CAD build for the part. Positions are in the model's coordinates, mm. Face numbers are marked on the shaded views. Round coordinates to 2 decimals unless told otherwise and drop trailing zeros. Order: outer loops, then holes, each group sorted by start corner. A loop starts at its lowest first (then second) coordinate and runs counter-clockwise, first axis right, second up. Notation, with made-up numbers: M 80,-39 L 137,-39 A21 cw 137,-13 Z; hole C 0,87.25 d6. An arc over 180 degrees is marked long. Answer as a JSON object with one key per item and string values. Group by question number.
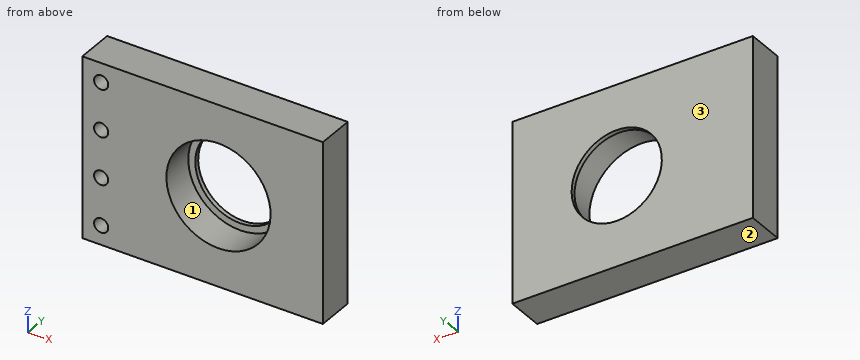
```python
from build123d import *

# Parameters (mm, degrees)
SKETCH1_W          = 50.8
SKETCH1_H          = 38.1
BODY_DEPTH         = 7.9375
SKETCH_1_R         = 9.525
THRU_HOLE_DEPTH    = 33.727150903
SKETCH4_R          = 10.9982
BEARING_BORE_DEPTH = 7.0104
SKETCH5_R          = 1.4986
DOWEL_HOLES_DEPTH  = 6.5


with BuildPart() as part:
    # Sketch1 → Body (new body)
    with BuildSketch(Plane(origin=(0, 0, 0), x_dir=(1, 0, 0), z_dir=(0, 1, 0))):
        Rectangle(SKETCH1_W, SKETCH1_H)
    extrude(amount=BODY_DEPTH)

    # Sketch 1 → Thru Hole (cut, through all)
    with BuildSketch(Plane.XZ):
        with Locations(Location((3.3528, 0, 0), (0, 0, 270))):
            Circle(SKETCH_1_R)
    extrude(amount=-THRU_HOLE_DEPTH, mode=Mode.SUBTRACT)

    # Sketch4 → Bearing Bore (cut)
    with BuildSketch(Plane.XZ):
        with Locations(Location((3.3528, 0, 0), (0, 0, 270))):
            Circle(SKETCH4_R)
    extrude(amount=-BEARING_BORE_DEPTH, mode=Mode.SUBTRACT)

    # Sketch5 → Dowel Holes (cut)
    with BuildSketch(Plane.XZ):
        with Locations(Location((-21.4249, 14.986, 0), (0, 0, 270))):
            Circle(SKETCH5_R)
        with Locations(Location((-21.4249, 4.995333333, 0), (0, 0, 270))):
            Circle(SKETCH5_R)
        with Locations(Location((-21.4249, -14.986, 0), (0, 0, 270))):
            Circle(SKETCH5_R)
        with Locations(Location((-21.4249, -4.995333333, 0), (0, 0, 270))):
            Circle(SKETCH5_R)
    extrude(amount=-DOWEL_HOLES_DEPTH, mode=Mode.SUBTRACT)


solid = part.part
```
Item 1: Cut at B-B, the plane x = 2. Give the cut face in (y, z).
Item 2: Two-plate mould, pull along Z, no slides. Class the marked faces 1, 2 and 3: +Z half, -Z half, draft (parallel to the pull), parting line (faces both ways), or undercut.
Item 3: Cut at D-D, the plane z = -14. Give the cut face in (x, y), and give its area (3 significant figures).
Item 4: Flat gauge pins, fed straight in: pin 1 Ø1.5 at (x, z) = (-21, -5.5) entering from -Y; pin 2 Ø2 at (x, z) = (13, 2) entering from -Y. Where does each tip first touch, or does it go through?
Item 5: Cut at A-A, the plane z = 0. Give the cut face in (x, y).
Item 6: Cut at C-C, the plane y = 2. Give the cut face in (x, z).
Item 7: Drill centre lines: line 1 (X direction, y = 1, z = -15); line 2 (X direction, y = 6.25, z = -4); line 3 (X direction, y = 1.25, z = -2). Where is each one in solid material? Low to high. Write a range as [from, to].
Response values:
{
 "1": {"outline": "M 0,-19.05 L 7.94,-19.05 L 7.94,-9.43 L 7.01,-9.43 L 7.01,-10.91 L 0,-10.91 Z; M 0,10.91 L 7.01,10.91 L 7.01,9.43 L 7.94,9.43 L 7.94,19.05 L 0,19.05 Z"},
 "2": {"face 1": "undercut", "face 2": "-Z half", "face 3": "draft"},
 "3": {"outline": "M -25.4,0 L -22.55,0 L -22.55,6.5 L -20.3,6.5 L -20.3,0 L 25.4,0 L 25.4,7.94 L -25.4,7.94 Z", "area": "389 mm^2"},
 "4": {"pin 1": "y = 6.5", "pin 2": "y = 7.01"},
 "5": {"outline": "M -25.4,0 L -7.65,0 L -7.65,7.01 L -6.17,7.01 L -6.17,7.94 L -25.4,7.94 Z; M 12.88,7.01 L 14.35,7.01 L 14.35,0 L 25.4,0 L 25.4,7.94 L 12.88,7.94 Z"},
 "6": {"outline": "M -25.4,-19.05 L 25.4,-19.05 L 25.4,19.05 L -25.4,19.05 Z; hole C -21.42,-14.99 d3; hole C -21.42,-5 d3; hole C -21.42,5 d3; hole C -21.42,14.99 d3; hole C 3.35,0 d22"},
 "7": {"line 1": "[-25.4, -22.92], [-19.93, 25.4]", "line 2": "[-25.4, -22.55], [-20.3, -6.89], [13.6, 25.4]", "line 3": "[-25.4, -7.46], [14.17, 25.4]"}
}
